```python
from build123d import *

# Parameters (mm, degrees)
SKETCH1_R           = 57.15
BOSS_EXTRUDE1_DEPTH = 177.8
CUT_EXTRUDE1_DEPTH  = 196.30766754
SHELL1_START        = 12.7
SHELL1_DEPTH        = 165.1


# Read off the part's stored shape, not the designer's step: Shell1
with BuildPart() as part:
    # Sketch1 → Boss-Extrude1 (new body)
    with BuildSketch(Plane(origin=(0, 0, 0), x_dir=(1, 0, 0), z_dir=(0, 1, 0))):
        with Locations(Location((0, 0, 0), (0, 0, 270))):
            Circle(SKETCH1_R)
    extrude(amount=BOSS_EXTRUDE1_DEPTH)

    # Sketch2 → Cut-Extrude1 (cut, through all)
    with BuildSketch(Plane(origin=(0, 177.8, 0), x_dir=(1, 0, 0), z_dir=(0, 1, 0))):
        Polygon((42.597094971, 323.940863218), (42.597094971, 38.1), (42.597094971, -38.1), (42.597094971, -323.940863218), (614.278821408, -323.940863218), (614.278821408, 323.940863218), align=None)
    extrude(amount=-CUT_EXTRUDE1_DEPTH, mode=Mode.SUBTRACT)

    # Shell1 outline → Shell1 (cut)
    with BuildSketch(Plane(origin=(0, 0, 0), x_dir=(1, 0, 0), z_dir=(0, 1, 0)).offset(SHELL1_START)):
        with BuildLine():
            ThreePointArc((17.197094971, 51.831573626), (-54.61, 0), (17.197094971, -51.831573626))
            Line((17.197094971, -51.831573626), (17.197094971, 51.831573626))
        make_face()
    extrude(amount=SHELL1_DEPTH, mode=Mode.SUBTRACT)


solid = part.part
```
Input: part model. Units: mm. Frame: model coordinates. A direction names the side the tool comes from. Give positions to 0.01 mm unless a question says otherwise; leave off trailing zeros. Order: outer loops, then holes, each group sorted by start corner. A loop starts at its lowest first (then second) coordinate and runs counter-clockwise, first axis right, second up. Notation, with made-up numbers: (28, 1.25) - (71, 1.25) arc R26 ccw to (71, 34.25) - close; hole circle Ø11 at (24.5, 8). An arc over 180 degrees is marked (long way). Put each result on its own line as item: value.
Item 1: Access query for faces 1 (the flat face through (-11, 12.7, -1)), 2 (the flat face through (42.597, 90, -1)). Directions: +Z, -Z, +X, -X, +Y, -Y. A direction counts if a zero-diameter tool reaches every point of the face in a straight line with its end or side. Return the directions, or none.
Found:
face 1: +Y
face 2: +Z, -Z, +X, +Y, -Y
Item 2: Section query A-A, the plane z = 0. Return loops of the section in (x, y), then the cut area to 3 significant figures.
Found:
outline: (-57.15, 0) - (42.6, 0) - (42.6, 177.8) - (17.2, 177.8) - (17.2, 12.7) - (-54.61, 12.7) - (-54.61, 177.8) - (-57.15, 177.8) - close
area: 5,880 mm^2
Item 3: Section query B-B, the plane x = 0. Return loops of the section in (y, z), then the cut area to 3 significant figures.
Found:
outline: (0, -57.15) - (177.8, -57.15) - (177.8, -54.61) - (12.7, -54.61) - (12.7, 54.61) - (177.8, 54.61) - (177.8, 57.15) - (0, 57.15) - close
area: 2,290 mm^2
Item 4: Ray query, L1, parallel to Z at x = 0, y = 130; L2, parallel to X at y = 122, z = 0; L3, parallel to Y at x = -5, z = -6. Return the intervals inside material, ascending. Write a range as from..to.
Found:
L1: z = -57.15..-54.61, 54.61..57.15
L2: x = -57.15..-54.61, 17.2..42.6
L3: y = 0..12.7
Item 5: Draft query along X for faces 3 (the cylindrical face through (-57.117, 87.655, -1.929)), 4 (the flat face through (-7, 0, -1)), 5 (the cylindrical face through (-54.59, 94.09, -1.45)). Return one class per face: +X half, -X half, draft (parallel to the pull), parting line (faces both ways), or undercut.
Found:
face 3: parting line
face 4: draft
face 5: undercut
Item 6: Section query D-D, the plane x = 28.5. Return loops of the section in (y, z), then the cut area to 3 significant figures.
Found:
outline: (0, -49.54) - (177.8, -49.54) - (177.8, 49.54) - (0, 49.54) - close
area: 17,600 mm^2
Item 7: Section query C-C, the plane y = 58. Return loops of the section in (x, z), then the cut area to 3 significant figures.
Found:
outline: (42.6, -38.1) - (42.6, 38.1) arc R57.15 ccw (long way) to start; hole (17.2, -51.83) - (17.2, 51.83) arc R54.61 ccw (long way) to start
area: 2,970 mm^2
Item 8: Contact query for flat-ended pins moving along their axis: pin 1 (10 mm diameter, centred on y = 114.5, z = -40, fed in from -X); pin 2 (12 mm diameter, centred on x = -26.5, y = 132.5, fed in from +Z); pin 3 (4 mm diameter, centred on x = 20, y = 28, fed in from +Z). Output: stop coordinate, or through.
Found:
pin 1: stops at x = -45.18
pin 2: stops at z = 53.35
pin 3: stops at z = 54.24
